Source: CAD feature listing. Evaluate the final solid. Frame: model axes, mm. A direction names the side the tool comes from. Give positions to 0.01 mm unless a question says otherwise; leave off trailing zeros. Write each loop counter-clockwise with the first axis right and the second up, starting at its lowest first coordinate (ties: lowest second). Pieces come first, ordered by that corner, then holes. Notation, with made-up numbers: M 38.5,43.25 L 46.5,43.25 A10 cw 46.5,48.25 Z; hole C 68,60.5 d9. An arc over 180 degrees is marked long. Answer as a JSON object with one key per item and string values. Group by question number.
```python
from build123d import *

# Parameters (mm, degrees)
F1_DEPTH = 25
F2_DEPTH = 25
F5_DEPTH = 4


with BuildPart() as f1:
    # F0 (on Front) → F1 (new body)
    with BuildSketch(Plane.XZ):
        Polygon((-67.6198684814, 0), (0, 0), (-41.0613296764, 63.8877525926), (-157.4556678534, 244.9869215488), (-205.308600446, 214.2313391182), align=None)
    extrude(amount=F1_DEPTH)

    # F0 (on Front) → F2 (join)
    with BuildSketch(Plane.XZ):
        Polygon((-41.0613296764, 63.8877525926), (0, 0), (281.2067568302, 0), (281.2067568302, 63.8877525926), align=None)
    extrude(amount=F2_DEPTH)

    # F4 (on offset) → F5 (join)
    with BuildSketch(Plane.XZ.offset(25)):
        Polygon((0, 0), (0, 63.8877525926), (-108.6811981577, 63.8877525926), (-67.6198684814, 0), align=None)
    extrude(amount=F5_DEPTH)


solid = f1.part
```
(1) Ray query, L1, parallel to Z at x = 114, y = -15.5; L2, parallel to Y at x = 21, z = 52.5; L3, parallel to X at y = -8.5, z = 145. Return the intervals inside material, ascending. Write a range as [from, to].
(2) Section D-D, the plane z = 153.5. Return loops of the section in (x, y), plus the area to 3 significant figures.
(3) Section C-C, the plane x = -13. Return loops of the section in (y, z).
(4) Contact query for flat-ended pins moving along their axis: pin 1 Ø2 at (x, y) = (192.5, -25.5) entering from +Z; pin 2 Ø4 at (y, z) = (-18.5, 119.5) entering from +X; pin 3 Ø10 at (x, y) = (-145, -12.5) entering from -Z. Output: stop coordinate, or through.
(5) Access query for faces 1 (the flat face through (19, 0, 50)), 2 (the flat face through (139, -25, 32)), 3 (the flat face through (-124, -25, 156)). Directions: +Z, -Z, +X, -X, +Y, -Y. A direction counts if a zero-diameter tool reaches every point of the face in a straight line with its end or side. Return the directions, or none.
(6) Section A-A, the plane y = -7. Return loops of the section in (x, z), plus the area to 3 significant figures.
(7) Section B-B, the plane z = 38. Return loops of the section in (x, y), plus the area to 3 significant figures.
Reported:
{
 "1": {"L1": "z = [0, 63.89]", "L2": "y = [-25, 0]", "L3": "x = [-160.81, -93.19]"},
 "2": {"outline": "M -166.28,-25 L -98.66,-25 L -98.66,0 L -166.28,0 Z", "area": "1,690 mm2"},
 "3": {"outline": "M -29,0 L 0,0 L 0,63.89 L -29,63.89 Z"},
 "4": {"pin 1": "stops at z = 63.89", "pin 2": "stops at x = -75.52", "pin 3": "stops at z = 112.62"},
 "5": {"face 1": "+Z, -Z, +X, -X, +Y", "face 2": "+Z, -Z, +X, -Y", "face 3": "+Z, +X, -X, -Y"},
 "6": {"outline": "M -205.31,214.23 L -67.62,0 L 281.21,0 L 281.21,63.89 L -41.06,63.89 L -157.46,244.99 Z", "area": "34,800 mm2"},
 "7": {"outline": "M -92.04,-29 L 0,-29 L 0,-25 L 281.21,-25 L 281.21,0 L -92.04,0 Z", "area": "9,700 mm2"}
}
